Design review of the part built by this model. Coordinates are the model's own, in mm. A direction names the side the tool comes from. Give positions to 0.01 mm unless a question says otherwise; leave off trailing zeros. Order: outer loops, then holes, each group sorted by start corner. A loop starts at its lowest first (then second) coordinate and runs counter-clockwise, first axis right, second up. Notation, with made-up numbers: (62, 88) -> (109, 88) arc R14 ccw to (109, 115) -> close; hole circle Ø5 at (5.5, 23). An arc over 180 degrees is marked (long way). One line per item, written item: value. Start each with the question number.
1) For pin 1 (5 mm diameter, centred on x = 25.4, y = 50.8, fed in from -Z); pin 2 (3.5 mm diameter, centred on x = 25.4, y = 41.275, fed in from -Z) (3 decimals), all flat-tipped, find the tip position at first contact; note any pin that passes through.
2) Tool access review of faces 4 (the face through (0, 576, -13)), 5 (the face through (26, 576, -3.175)): name each direction out of +Z, -Z, +X, -X, +Y, -Y from which nothing blocks a thin tool from reaching the whole face with its end or side.
3) Wall thickness on line 1 along X through (y, z) = (297, -8.25) (3 decimals); line 2 along X through (y, z) = (457.2, -1.75) (3 decimals); line 3 along Z through (x, y) = (14.5, 254.5) (3 decimals): over which ranges is each line inside the solid? List them lowest first. Write a range as from..to.
4) The part is to be moulded in two halves that separate along X. For faces 1 (the face through (47.625, 576, -14)), 2 (the face through (27, 1168.4, -2)), 3 (the face through (50.8, 576, -13)), say which applies: released by +X, released by -X, zero draft, split by the parting line, or undercut.
5) Consider section B-B (y = 987.5). State the section outline as (x, z) points (3 decimals).
6) Consider section A-A (z = -12.5). State the section outline as (x, y) points (3 decimals).
from build123d import *

# Parameters (mm, degrees)
BOSS_EXTRUDE1_DEPTH = 1168.4
CUT_EXTRUDE1_REACH  = 27.4
SKETCH2_R           = 3.175
CUT_EXTRUDE2_REACH  = 27.4
SKETCH4_R           = 1.5875


with BuildPart() as part:
    # Sketch1 → Boss-Extrude1 (new body)
    with BuildSketch(Plane(origin=(0, 0, 0), x_dir=(1, 0, 0), z_dir=(0, 1, 0))):
        Polygon((3.175, 3.175), (3.175, 25.4), (0, 25.4), (0, 0), (50.8, 0), (50.8, 25.4), (47.625, 25.4), (47.625, 3.175), align=None)
    extrude(amount=BOSS_EXTRUDE1_DEPTH)

    # Sketch2 → Cut-Extrude1 (cut, up to next)
    with BuildSketch(Plane.XY, mode=Mode.PRIVATE) as cut_extrude1_sk1:
        with Locations((25.4, 50.8)):
            Circle(SKETCH2_R)
    cut_extrude1_tool1 = extrude(cut_extrude1_sk1.sketch, amount=-CUT_EXTRUDE1_REACH, mode=Mode.PRIVATE) & part.part
    add(cut_extrude1_tool1.solids().sort_by_distance((25.4, 50.8, 0))[0], mode=Mode.SUBTRACT)
    # Sketch2 → Cut-Extrude1 (cut, up to next)
    with BuildSketch(Plane.XY, mode=Mode.PRIVATE) as cut_extrude1_sk2:
        with Locations((25.4, 152.4)):
            Circle(SKETCH2_R)
    cut_extrude1_tool2 = extrude(cut_extrude1_sk2.sketch, amount=-CUT_EXTRUDE1_REACH, mode=Mode.PRIVATE) & part.part
    add(cut_extrude1_tool2.solids().sort_by_distance((25.4, 152.4, 0))[0], mode=Mode.SUBTRACT)
    # Sketch2 → Cut-Extrude1 (cut, up to next)
    with BuildSketch(Plane.XY, mode=Mode.PRIVATE) as cut_extrude1_sk3:
        with Locations((25.4, 254)):
            Circle(SKETCH2_R)
    cut_extrude1_tool3 = extrude(cut_extrude1_sk3.sketch, amount=-CUT_EXTRUDE1_REACH, mode=Mode.PRIVATE) & part.part
    add(cut_extrude1_tool3.solids().sort_by_distance((25.4, 254, 0))[0], mode=Mode.SUBTRACT)
    # Sketch2 → Cut-Extrude1 (cut, up to next)
    with BuildSketch(Plane.XY, mode=Mode.PRIVATE) as cut_extrude1_sk4:
        with Locations((25.4, 355.6)):
            Circle(SKETCH2_R)
    cut_extrude1_tool4 = extrude(cut_extrude1_sk4.sketch, amount=-CUT_EXTRUDE1_REACH, mode=Mode.PRIVATE) & part.part
    add(cut_extrude1_tool4.solids().sort_by_distance((25.4, 355.6, 0))[0], mode=Mode.SUBTRACT)
    # Sketch2 → Cut-Extrude1 (cut, up to next)
    with BuildSketch(Plane.XY, mode=Mode.PRIVATE) as cut_extrude1_sk5:
        with Locations((25.4, 457.2)):
            Circle(SKETCH2_R)
    cut_extrude1_tool5 = extrude(cut_extrude1_sk5.sketch, amount=-CUT_EXTRUDE1_REACH, mode=Mode.PRIVATE) & part.part
    add(cut_extrude1_tool5.solids().sort_by_distance((25.4, 457.2, 0))[0], mode=Mode.SUBTRACT)
    # Sketch2 → Cut-Extrude1 (cut, up to next)
    with BuildSketch(Plane.XY, mode=Mode.PRIVATE) as cut_extrude1_sk6:
        with Locations((25.4, 558.8)):
            Circle(SKETCH2_R)
    cut_extrude1_tool6 = extrude(cut_extrude1_sk6.sketch, amount=-CUT_EXTRUDE1_REACH, mode=Mode.PRIVATE) & part.part
    add(cut_extrude1_tool6.solids().sort_by_distance((25.4, 558.8, 0))[0], mode=Mode.SUBTRACT)
    # Sketch2 → Cut-Extrude1 (cut, up to next)
    with BuildSketch(Plane.XY, mode=Mode.PRIVATE) as cut_extrude1_sk7:
        with Locations((25.4, 660.4)):
            Circle(SKETCH2_R)
    cut_extrude1_tool7 = extrude(cut_extrude1_sk7.sketch, amount=-CUT_EXTRUDE1_REACH, mode=Mode.PRIVATE) & part.part
    add(cut_extrude1_tool7.solids().sort_by_distance((25.4, 660.4, 0))[0], mode=Mode.SUBTRACT)
    # Sketch2 → Cut-Extrude1 (cut, up to next)
    with BuildSketch(Plane.XY, mode=Mode.PRIVATE) as cut_extrude1_sk8:
        with Locations((25.4, 762)):
            Circle(SKETCH2_R)
    cut_extrude1_tool8 = extrude(cut_extrude1_sk8.sketch, amount=-CUT_EXTRUDE1_REACH, mode=Mode.PRIVATE) & part.part
    add(cut_extrude1_tool8.solids().sort_by_distance((25.4, 762, 0))[0], mode=Mode.SUBTRACT)
    # Sketch2 → Cut-Extrude1 (cut, up to next)
    with BuildSketch(Plane.XY, mode=Mode.PRIVATE) as cut_extrude1_sk9:
        with Locations((25.4, 863.6)):
            Circle(SKETCH2_R)
    cut_extrude1_tool9 = extrude(cut_extrude1_sk9.sketch, amount=-CUT_EXTRUDE1_REACH, mode=Mode.PRIVATE) & part.part
    add(cut_extrude1_tool9.solids().sort_by_distance((25.4, 863.6, 0))[0], mode=Mode.SUBTRACT)
    # Sketch2 → Cut-Extrude1 (cut, up to next)
    with BuildSketch(Plane.XY, mode=Mode.PRIVATE) as cut_extrude1_sk10:
        with Locations((25.4, 965.2)):
            Circle(SKETCH2_R)
    cut_extrude1_tool10 = extrude(cut_extrude1_sk10.sketch, amount=-CUT_EXTRUDE1_REACH, mode=Mode.PRIVATE) & part.part
    add(cut_extrude1_tool10.solids().sort_by_distance((25.4, 965.2, 0))[0], mode=Mode.SUBTRACT)
    # Sketch2 → Cut-Extrude1 (cut, up to next)
    with BuildSketch(Plane.XY, mode=Mode.PRIVATE) as cut_extrude1_sk11:
        with Locations((25.4, 1066.8)):
            Circle(SKETCH2_R)
    cut_extrude1_tool11 = extrude(cut_extrude1_sk11.sketch, amount=-CUT_EXTRUDE1_REACH, mode=Mode.PRIVATE) & part.part
    add(cut_extrude1_tool11.solids().sort_by_distance((25.4, 1066.8, 0))[0], mode=Mode.SUBTRACT)

    # Sketch4 → Cut-Extrude2 (cut, up to next)
    with BuildSketch(Plane.XY, mode=Mode.PRIVATE) as cut_extrude2_sk1:
        with Locations((25.4, 41.275)):
            Circle(SKETCH4_R)
    cut_extrude2_tool1 = extrude(cut_extrude2_sk1.sketch, amount=-CUT_EXTRUDE2_REACH, mode=Mode.PRIVATE) & part.part
    add(cut_extrude2_tool1.solids().sort_by_distance((25.4, 41.275, 0))[0], mode=Mode.SUBTRACT)
    # Sketch4 → Cut-Extrude2 (cut, up to next)
    with BuildSketch(Plane.XY, mode=Mode.PRIVATE) as cut_extrude2_sk2:
        with Locations((25.4, 12.7)):
            Circle(SKETCH4_R)
    cut_extrude2_tool2 = extrude(cut_extrude2_sk2.sketch, amount=-CUT_EXTRUDE2_REACH, mode=Mode.PRIVATE) & part.part
    add(cut_extrude2_tool2.solids().sort_by_distance((25.4, 12.7, 0))[0], mode=Mode.SUBTRACT)


solid = part.part
Checked values:
1. pin 1: passes through
1. pin 2: stops at z = -3.175
2. face 4: +Z, -Z, -X, +Y, -Y
2. face 5: -Z, +Y, -Y
3. line 1: x = 0..3.175, 47.625..50.8
3. line 2: x = 0..22.225, 28.575..50.8
3. line 3: z = -3.175..0
4. face 1: undercut
4. face 2: zero draft
4. face 3: released by +X
5. outline: (0, -25.4) -> (3.175, -25.4) -> (3.175, -3.175) -> (47.625, -3.175) -> (47.625, -25.4) -> (50.8, -25.4) -> (50.8, 0) -> (0, 0) -> close
6. outline: (0, 0) -> (3.175, 0) -> (3.175, 1168.4) -> (0, 1168.4) -> close; (47.625, 0) -> (50.8, 0) -> (50.8, 1168.4) -> (47.625, 1168.4) -> close
